from build123d import *

# Parameters (mm, degrees)
F0_R     = 27.251254
F1_DEPTH = 47.244
F2_DEPTH = 12.7
F4_DEPTH = 25.4
F6_DEPTH = 51.905433


with BuildPart() as f1:
    # F0 (on Top) → F1 (new body)
    with BuildSketch(Plane.XY):
        with BuildLine():
            ThreePointArc((-29.068472, -26.332406), (14.11109, -36.595749), (39.222081, 0))
            ThreePointArc((39.222081, 0), (14.11109, 36.595749), (-29.068472, 26.332406))
            ThreePointArc((-29.068472, 26.332406), (-39.222081, 0), (-29.068472, -26.332406))
        make_face()
        Circle(F0_R, mode=Mode.SUBTRACT)
    extrude(amount=F1_DEPTH)

    # F0 (on Top) → F2 (join)
    with BuildSketch(Plane.XY):
        with BuildLine():
            ThreePointArc((-29.068472, -26.332406), (-39.222081, 0), (-29.068472, 26.332406))
            Line((-29.068472, 26.332406), (-93.851398, 26.332406))
            Line((-93.851398, 26.332406), (-93.851398, -26.332406))
            Line((-93.851398, -26.332406), (-29.068472, -26.332406))
        make_face()
    extrude(amount=F2_DEPTH)

    # F3 (on face) → F4 (join)
    with BuildSketch(Plane.XY.offset(12.7)):
        with BuildLine():
            ThreePointArc((-37.115086, -12.682351), (-39.222081, 0), (-37.115086, 12.682351))
            Line((-37.115086, 12.682351), (-64.119155, 12.682351))
            Line((-64.119155, 12.682351), (-64.119155, -12.682351))
            Line((-64.119155, -12.682351), (-37.115086, -12.682351))
        make_face()
    extrude(amount=F4_DEPTH)

    # F5 (on face) → F6 (cut, through all)
    with BuildSketch(Plane.XZ.offset(12.682351)):
        Polygon((-64.119155, 12.7), (-37.115086, 38.1), (-64.119155, 38.1), align=None)
    extrude(amount=-F6_DEPTH, mode=Mode.SUBTRACT)


solid = f1.part
Read the model definition and answer for the solid it produces. Units are mm, in the model's axes. A direction names the side the tool comes from. Round coordinates to 2 decimals unless told otherwise and drop trailing zeros. Order: outer loops, then holes, each group sorted by start corner. A loop starts at its lowest first (then second) coordinate and runs counter-clockwise, first axis right, second up.
1) Straight lines are drawn through the part: L1, parallel to Y at x = 0, z = 26; L2, parallel to Z at x = -38, y = 21.5; L3, parallel to Y at x = -6, z = 44. For each, find the intervals that lie inside material, in ascending order.
2) The mould has two halves that part along Y. Classify faces 1 (the face through (-47, 12.682, 22)), 2 (the face through (-5.908, -26.603, 23.291)), 3 (the face through (-45, -12.682, 20)), 4 (the face through (-93.851, 0, 6)): released by +Y, released by -Y, zero draft, split by the parting line, or undercut.
3) For faces 5 (the face through (-61, 26.332, 6)), 6 (the face through (-69, 0, 12.7)), 7 (the face through (-27, -8, 47.244)), 8 (the face through (-62, -26.332, 6)), 9 (the face through (-28, 1, 0)), determine the directions among +Z, -Z, +X, -X, +Y, -Y from which every point of the face is accessible in a straight line to the end or side of a thin tool.
4) The part is cut by section A-A on x = 0. Write down the section's boundary in (y, z).
5) Flat-ended cylindrical pins translate along their axes: pin 1 (8 mm diameter, centred on x = 16.5, z = 27, fed in from +Y); pin 2 (7.5 mm diameter, centred on x = -46.5, z = 21, fed in from -Y); pin 3 (2.5 mm diameter, centred on x = -38, y = -6, fed in from -Z); pin 4 (4 mm diameter, centred on y = 21.5, z = 39, fed in from -X). Find the tip coordinate at first contact, or state that the pin passes through.
6) The part is cut by section D-D on x = -34. Write down the section's boundary in (y, z), plus the area to 3 significant figures.
7) The part is cut by section B-B on y = 2.5. Write down the section's boundary in (x, z), plus the area to 3 significant figures.
8) The part is cut by section C-C on z = 39.5. Write down the section's boundary in (x, y), plus the area to 3 significant figures.
Resolved:
1. L1: y = -39.22 to -27.25, 27.25 to 39.22
1. L2: z = 0 to 12.7
1. L3: y = -38.76 to -26.58, 26.58 to 38.76
2. face 1: released by +Y
2. face 2: undercut
2. face 3: released by -Y
2. face 4: zero draft
3. face 5: +Z, -Z, -X, +Y
3. face 6: +Z, -X
3. face 7: +Z, +X, -X, +Y, -Y
3. face 8: +Z, -Z, -X, -Y
3. face 9: -Z, +X, -X, +Y, -Y
4. outline: (-39.22, 0) - (-27.25, 0) - (-27.25, 47.24) - (-39.22, 47.24) - close; (27.25, 0) - (39.22, 0) - (39.22, 47.24) - (27.25, 47.24) - close
5. pin 1: stops at y = 37.18
5. pin 2: stops at y = -12.68
5. pin 3: stops at z = 0
5. pin 4: stops at x = -34.03
6. outline: (-26.33, 0) - (26.33, 0) - (26.33, 12.7) - (19.55, 12.7) - (19.55, 47.24) - (-19.55, 47.24) - (-19.55, 12.7) - (-26.33, 12.7) - close
6. area: 2,020 mm2
7. outline: (-93.85, 0) - (-27.14, 0) - (-27.14, 47.24) - (-39.14, 47.24) - (-39.14, 38.1) - (-37.12, 38.1) - (-64.12, 12.7) - (-93.85, 12.7) - close; (27.14, 0) - (39.14, 0) - (39.14, 47.24) - (27.14, 47.24) - close
7. area: 2,120 mm2
8. outline: (-29.07, -26.33) arc R39.22 ccw to (39.22, 0) arc R39.22 ccw to (-29.07, 26.33) arc R39.22 ccw to start; hole circle Ø54.5 at (0, 0)
8. area: 2,500 mm2
